Can you work these out from the model? Positions are in its coordinate system, mm. A direction names the side the tool comes from. Coordinates: 2 decimals unless noted, no trailing zeros. Order: outer loops, then holes, each group sorted by start corner. A loop starts at its lowest first (then second) coordinate and runs counter-clockwise, first axis right, second up. Notation, with made-up numbers: (35.5, -1.5) -> (83.5, -1.5) arc R20 ccw to (83.5, 16.5) -> close; hole circle Ø6 at (26.5, 87.25). An arc over 180 degrees is marked (long way). Write item = value, one per line.
```python
from build123d import *

# Parameters (mm, degrees)
SKETCH061_W     = 24.5
SKETCH061_H     = 20
PAD029_DEPTH    = 24
SKETCH062_W     = 24.5
SKETCH062_H     = 10.5
POCKET039_DEPTH = 6
CHAMFER023_SIZE = 3
SKETCH063_R     = 1
POCKET040_DEPTH = 24.001
CHAMFER025_SIZE = 3


with BuildPart() as part:
    # Sketch061 → Pad029 (new body)
    with BuildSketch(Plane.XY):
        with Locations((-183.55, 206.2)):
            Rectangle(SKETCH061_W, SKETCH061_H)
    extrude(amount=PAD029_DEPTH)

    # Sketch062 (on Face6 of Pad029) → Pocket039 (cut)
    with BuildSketch(Plane.XY.offset(24)):
        with Locations((-183.55, 201.45)):
            Rectangle(SKETCH062_W, SKETCH062_H)
    extrude(amount=-POCKET039_DEPTH, mode=Mode.SUBTRACT)

    # Chamfer023
    chamfer023_edges = [part.edges().sort_by_distance(p)[0] for p in [
        (-171.3, 201.45, 18),
    ]]
    chamfer(chamfer023_edges, length=CHAMFER023_SIZE)

    # Sketch063 (on Face7 of Chamfer023) → Pocket040 (cut, through all)
    with BuildSketch(Plane.XY.offset(24)):
        with Locations((-189.55, 210.725281)):
            Circle(SKETCH063_R)
        with Locations((-177.55, 210.725281)):
            Circle(SKETCH063_R)
    extrude(amount=-POCKET040_DEPTH, mode=Mode.SUBTRACT)

    # Chamfer025
    chamfer025_edges = [part.edges().sort_by_distance(p)[0] for p in [
        (-171.3, 206.2, 0),
    ]]
    chamfer(chamfer025_edges, length=CHAMFER025_SIZE)


with BuildPart() as part_1:
    # Body022 placement: moved
    add(part.part.moved(Location((0, 0, -8.6))))


solid = part_1.part
```
Item 1: For faces 4 (the flat face through (-172.8, 201.4, 7.9)), 5 (the flat face through (-185, 202, 9.4)), 6 (the flat face through (-172.8, 206.1, -7.1)), which set-ups out of +Z, -Z, +X, -X, +Y, -Y let a thin tool reach every point of the face, with its end or its side?
A:
face_4 = +Z, +X, -Y
face_5 = +Z, +X, -X, -Y
face_6 = -Z, +X, +Y, -Y
Item 2: If I drill on probe 1 along Y at (x, z) = (-177.55, -1.5); probe 2 along Y at (x, z) = (-189.55, 10); probe 3 along Z at (x, y) = (-175.5, 202.25), over which ranges is the centre line in solid material (lowest first)?
A:
probe_1 = 196.2 to 209.73, 211.73 to 216.2
probe_2 = 206.7 to 209.73, 211.73 to 216.2
probe_3 = -8.6 to 9.4
Item 3: If we mould it in two halves opening along Y, with no side actions, what happens to faces 1 (the cylindrical face through (-177.089, 209.838, 3.568)), 2 (the flat face through (-184, 216.2, 3)), 3 (the flat face through (-195.8, 206, 3))? For each: pulls with the +Y half, pulls with the -Y half, needs draft (parallel to the pull), parting line crosses it, or undercut.
A:
face_1 = undercut
face_2 = pulls with the +Y half
face_3 = needs draft
Item 4: I want a section at B-B, the plane z = 9. Please give me the cut outline in (x, y).
A:
outline = (-195.8, 196.2) -> (-173.9, 196.2) -> (-173.9, 206.7) -> (-171.3, 206.7) -> (-171.3, 216.2) -> (-195.8, 216.2) -> close; hole circle Ø2 at (-189.55, 210.73); hole circle Ø2 at (-177.55, 210.73)
Item 5: I want a section at C-C, the plane x = -175. Please give me the cut outline in (y, z).
A:
outline = (196.2, -8.6) -> (216.2, -8.6) -> (216.2, 15.4) -> (206.7, 15.4) -> (206.7, 9.4) -> (196.2, 9.4) -> close
Item 6: I want a section at D-D, the plane y = 199. Please give me the cut outline in (x, z).
A:
outline = (-195.8, -8.6) -> (-174.3, -8.6) -> (-171.3, -5.6) -> (-171.3, 6.4) -> (-174.3, 9.4) -> (-195.8, 9.4) -> close
Item 7: I want a section at A-A, the plane x = -189.55. Please give me the cut outline in (y, z).
A:
outline = (196.2, -8.6) -> (209.73, -8.6) -> (209.73, 15.4) -> (206.7, 15.4) -> (206.7, 9.4) -> (196.2, 9.4) -> close; (211.73, -8.6) -> (216.2, -8.6) -> (216.2, 15.4) -> (211.73, 15.4) -> close
Item 8: I'm going to push a flat-ended pin straight in: P1, Ø8.5, axis at x = -182, y = 202, coming from the +Z side. Where does the tip first touch, or does it pass through?
A:
P1 = 9.4
